Verification items for the finished model (mm, model axes). Face numbers are marked on the shaded views. A direction names the side the tool comes from. Round coordinates to 2 decimals unless told otherwise and drop trailing zeros. Loops run counter-clockwise (first coordinate to the right, second up) from the corner with the lowest first, then second, coordinate; pieces in that order, holes last. Notation, with made-up numbers: M 27.25,31.25 L 62.25,31.25 A28 ccw 62.25,63.25 Z; hole C -25,1 d3. An arc over 180 degrees is marked long. Answer as CSV lines item,"result".
```python
from build123d import *

# Parameters (mm, degrees)
BODY_DEPTH = 2.54
SKETCH2_R  = 1.143
FLAG_DEPTH = 7.62
SKETCH3_R  = 2.54
FEET_DEPTH = 1.778


with BuildPart() as part:
    # Sketch1 → body (new body)
    with BuildSketch(Plane(origin=(0, 0, 0), x_dir=(1, 0, 0), z_dir=(0, 1, 0))):
        Polygon((-8.348684361, -10.452067183), (-8.348684361, -4.102067183), (-1.998684361, -4.102067183), (-1.998684361, -10.452067183), (4.351315639, -10.452067183), (4.351315639, -16.802067183), (-1.998684361, -16.802067183), (-1.998684361, -23.152067183), (-8.348684361, -23.152067183), (-8.348684361, -16.802067183), (-14.698684361, -16.802067183), (-14.698684361, -10.452067183), align=None)
    extrude(amount=BODY_DEPTH)

    # Sketch2 → flag (add)
    with BuildSketch(Plane(origin=(0, 2.54, 0), x_dir=(1, 0, 0), z_dir=(0, 1, 0))):
        with Locations(Location((-5.173684361, -7.277067183, 0), (0, 0, 90))):
            Circle(SKETCH2_R)
        with Locations(Location((1.176315639, -13.627067183, 0), (0, 0, 90))):
            Circle(SKETCH2_R)
        with Locations(Location((-5.173684361, -19.977067183, 0), (0, 0, 90))):
            Circle(SKETCH2_R)
        with Locations(Location((-11.523684361, -13.627067183, 0), (0, 0, 90))):
            Circle(SKETCH2_R)
    extrude(amount=FLAG_DEPTH)

    # Sketch3 → feet (add)
    with BuildSketch(Plane(origin=(0, 10.16, 0), x_dir=(1, 0, 0), z_dir=(0, 1, 0))):
        with Locations(Location((-5.173684361, -7.277067183, 0), (0, 0, 270))):
            Circle(SKETCH3_R)
        with Locations(Location((-11.523684361, -13.627067183, 0), (0, 0, 270))):
            Circle(SKETCH3_R)
        with Locations(Location((-5.173684361, -19.977067183, 0), (0, 0, 270))):
            Circle(SKETCH3_R)
        with Locations(Location((1.176315639, -13.627067183, 0), (0, 0, 270))):
            Circle(SKETCH3_R)
    extrude(amount=FEET_DEPTH)


solid = part.part
```
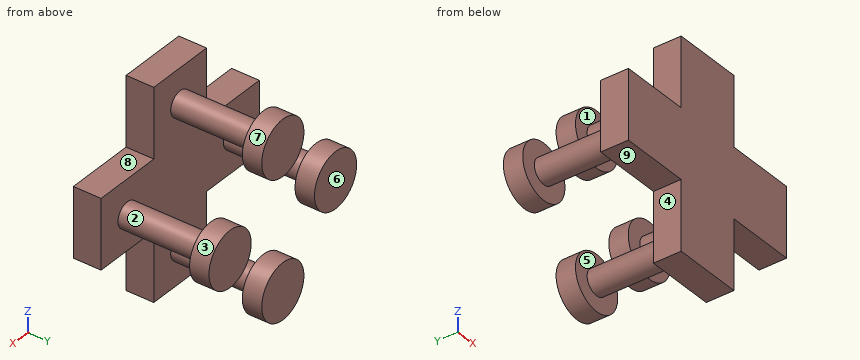
1) Section check C-C (x = -0.5). Record the cut outline in (y, z), plus the area to 3 significant figures.
Here are the results:
outline,"M 0,10.45 L 2.54,10.45 L 2.54,16.8 L 0,16.8 Z; M 10.16,11.72 L 11.94,11.72 L 11.94,15.54 L 10.16,15.54 Z"
area,"22.9 mm^2"
2) Section check D-D (y = 11). Record the cut outline in (x, z), plus the area to 3 significant figures.
Here are the results:
outline,"C -11.52,13.63 d5.08; C -5.17,7.28 d5.08; C -5.17,19.98 d5.08; C 1.18,13.63 d5.08"
area,"81.1 mm^2"
3) Draft check along X on the marked faces 1, 2, 3 and 4. Enter one of: +X half, -X half, draft (parallel to the pull), parting line (faces both ways), or undercut.
Here are the results:
face 1,"draft"
face 2,"undercut"
face 3,"undercut"
face 4,"-X half"
4) Section check A-A (y = 2). Record the cut outline in (x, z).
Here are the results:
outline,"M -14.7,10.45 L -8.35,10.45 L -8.35,4.1 L -2,4.1 L -2,10.45 L 4.35,10.45 L 4.35,16.8 L -2,16.8 L -2,23.15 L -8.35,23.15 L -8.35,16.8 L -14.7,16.8 Z"
5) Material ranges on probe 1 along Z at (x, y) = (-5.25, 7.5); probe 2 along Y at (x, z) = (2.75, 12); probe 3 along Y at (x, z) = (-1.25, 16.25), recorded low to high.
Here are the results:
probe 1,"z = 6.14 to 8.42, 18.84 to 21.12"
probe 2,"y = 0 to 2.54, 10.16 to 11.94"
probe 3,"y = 0 to 2.54"
6) Set-up check for the marked faces 5, 6, 7, 8 and 9: record each of +Z, -Z, +X, -X, +Y, -Y from which the full face is reachable in a straight line by a thin tool's end or side.
Here are the results:
face 5,"none"
face 6,"+Z, -Z, +X, -X, +Y"
face 7,"+Y"
face 8,"+Z, +X, +Y, -Y"
face 9,"-Z, -X, +Y, -Y"
7) Go/stop test with flat-tipped pins: pin 1 (0.8 mm diameter, centred on y = 0.5, z = 7.5, fed in from +X); pin 2 (2 mm diameter, centred on x = -10, y = 1, fed in from +Z); pin 3 (3 mm diameter, centred on x = -12, y = 1, fed in from -Z); pin 4 (1 mm diameter, centred on y = 4.5, z = 18, fed in from +X). Record where each tip stops, or that it passes through.
Here are the results:
pin 1,"stops at x = -2"
pin 2,"stops at z = 16.8"
pin 3,"stops at z = 10.45"
pin 4,"passes through"
8) Section check B-B (z = 7). Record the cut outline in (x, y).
Here are the results:
outline,"M -8.35,0 L -2,0 L -2,2.54 L -4.06,2.54 L -4.06,10.16 L -2.65,10.16 L -2.65,11.94 L -7.7,11.94 L -7.7,10.16 L -6.28,10.16 L -6.28,2.54 L -8.35,2.54 Z"
